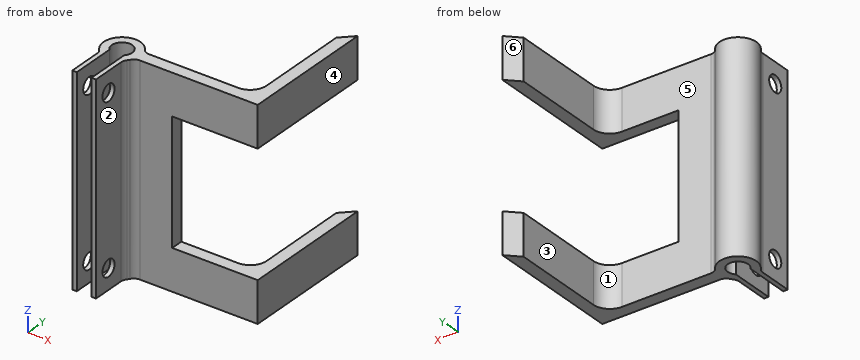
```python
from build123d import *

# Parameters (mm, degrees)
SKETCH_1_R          = 2.25
SKETCH_1_R_2        = 1.25
EXTRUDE_1_DEPTH     = 25
EXTRUDE_START       = -25
EXTRUDE_2_DEPTH     = 25
CUT_EXTRUDE_1_DEPTH = 25
SKETCH_4_W          = 0.55
SKETCH_4_H          = 25
EXTRUDE_3_DEPTH     = 2
EXTRUDE_4_DEPTH     = 25
FILLET_1_R          = 1
SKETCH_6_W          = 1.5
SKETCH_6_H          = 25
EXTRUDE_6_DEPTH     = 15
SKETCH_7_W          = 17.879358453
SKETCH_7_H          = 15
CUT_EXTRUDE_2_DEPTH = 50
FILLET_2_R          = 2
SKETCH_8_R          = 1
CUT_EXTRUDE_3_DEPTH = 10
CHAMFER_1_SIZE      = 1.5


with BuildPart() as part:
    # 草图1 → 凸台-拉伸1 (new body)
    with BuildSketch(Plane.XY):
        Circle(SKETCH_1_R)
        Circle(SKETCH_1_R_2, mode=Mode.SUBTRACT)
    extrude(amount=EXTRUDE_1_DEPTH)

    # 草图2 → 凸台-拉伸2 (add)
    with BuildSketch(Plane.XY.offset(25).offset(EXTRUDE_START)):
        with BuildLine():
            Line((-0.9, -4.25), (-0.9, -2.062159063))
            ThreePointArc((-0.9, -2.062159063), (-1.187355759, -1.911200225), (-1.45, -1.720465053))
            Line((-1.45, -1.720465053), (-1.45, -4.25))
            Line((-1.45, -4.25), (-0.9, -4.25))
        make_face()
        with BuildLine():
            ThreePointArc((1.45, -1.720465053), (1.187355759, -1.911200225), (0.9, -2.062159063))
            Line((0.9, -2.062159063), (0.9, -4.25))
            Line((0.9, -4.25), (1.45, -4.25))
            Line((1.45, -4.25), (1.45, -1.720465053))
        make_face()
    extrude(amount=EXTRUDE_2_DEPTH)

    # 草图3 → 切除-拉伸1 (cut)
    with BuildSketch(Plane.XY.offset(25)):
        Polygon((-0.9, -2.062159063), (-0.9, -0.608172981), (0.9, -0.572608175), (0.9, -2.062159063), (-0.22034315, -2.711539451), align=None)
    extrude(amount=-CUT_EXTRUDE_1_DEPTH, mode=Mode.SUBTRACT)

    # 草图4 → 凸台-拉伸3 (add)
    with BuildSketch(Plane.XZ.offset(4.25)):
        with Locations((1.175, 12.5)):
            Rectangle(SKETCH_4_W, SKETCH_4_H)
        with Locations((-1.175, 12.5)):
            Rectangle(SKETCH_4_W, SKETCH_4_H)
    extrude(amount=EXTRUDE_3_DEPTH)

    # 草图5 → 凸台-拉伸4 (add)
    with BuildSketch(Plane.XY.offset(25).offset(EXTRUDE_START)):
        with BuildLine():
            Line((2.121320344, 0.75), (17.121320344, 0.75))
            Line((17.121320344, 0.75), (17.121320344, -0.75))
            Line((17.121320344, -0.75), (2.121320344, -0.75))
            ThreePointArc((2.121320344, -0.75), (2.25, 0), (2.121320344, 0.75))
        make_face()
    extrude(amount=EXTRUDE_4_DEPTH)

    # 圆角1
    fillet_1_edges = [part.edges().sort_by_distance(p)[0] for p in [
        (-1.45, -1.720465053, 12.5),
        (1.45, -1.720465053, 12.5),
        (2.121320344, -0.75, 12.5),
        (2.121320344, 0.75, 12.5),
    ]]
    fillet(fillet_1_edges, radius=FILLET_1_R)

    # 草图6 → 凸台-拉伸6 (add)
    with BuildSketch(Plane(origin=(0, 0.75, 0), x_dir=(1, 0, 0), z_dir=(0, 1, 0))):
        with Locations((16.371320344, -12.5)):
            Rectangle(SKETCH_6_W, SKETCH_6_H)
    extrude(amount=EXTRUDE_6_DEPTH)

    # 草图7 → 切除-拉伸2 (cut, symmetric)
    with BuildSketch(Plane(origin=(0, 0.75, 0), x_dir=(1, 0, 0), z_dir=(0, 1, 0))):
        with Locations((15.621320344, -12.5)):
            Rectangle(SKETCH_7_W, SKETCH_7_H)
    extrude(amount=CUT_EXTRUDE_2_DEPTH, both=True, mode=Mode.SUBTRACT)

    # 圆角2
    fillet_2_edges = [part.edges().sort_by_distance(p)[0] for p in [
        (15.621320344, 0.75, 2.5),
        (15.621320344, 0.75, 22.5),
    ]]
    fillet(fillet_2_edges, radius=FILLET_2_R)

    # 草图8 → 切除-拉伸3 (cut)
    with BuildSketch(Plane.ZY.offset(1.45)):
        with Locations((2.5, -4.192707825)):
            Circle(SKETCH_8_R)
        with Locations((22.5, -4.192707825)):
            Circle(SKETCH_8_R)
    extrude(amount=-CUT_EXTRUDE_3_DEPTH, mode=Mode.SUBTRACT)

    # 倒角1
    chamfer_1_edges = [part.edges().sort_by_distance(p)[0] for p in [
        (15.621320344, 15.75, 2.5),
        (15.621320344, 15.75, 22.5),
    ]]
    chamfer(chamfer_1_edges, length=CHAMFER_1_SIZE - 0.0001)  # a hair under: the kernel refuses the full size


solid = part.part
```
Check sheet for the modelled part. Datum: model origin and axes. Units: mm. Face numbers are marked on the shaded views. A direction names the side the tool comes from. Round coordinates to 2 decimals unless told otherwise and drop trailing zeros. Order: outer loops, then holes, each group sorted by start corner. A loop starts at its lowest first (then second) coordinate and runs counter-clockwise, first axis right, second up.
1) Section check D-D (z = 17.75). Record the boundary of the cut face in (x, y).
2) Tool access check on the marked faces 1, 2 and 3. Record the directions out of +Z, -Z, +X, -X, +Y, -Y that give a thin tool (end or side, any length) a straight path to the whole face; none if there is none.
3) Section check C-C (x = 12). Record the boundary of the cut face in (y, z).
4) Mould release check, pull along X, two halves, no side actions. Record for the marked faces 4, 5 and 6: +X half, -X half, draft (parallel to the pull), parting line (faces both ways), or undercut.
5) Section check B-B (y = 0). Record the boundary of the cut face in (x, z), and give its area (3 significant figures).
6) Go/stop test with flat-tipped pins: pin 1 Ø2 at (x, y) = (0, 0) entering from +Z; pin 2 Ø3 at (x, z) = (5.5, 14.5) entering from +Y; pin 3 Ø2.5 at (y, z) = (10, 2.5) entering from -X; pin 4 Ø4.5 at (y, z) = (-4.5, 12.5) entering from -X. Record where each tip stops, or that it passes through.
7) Scan lines: line 1 (Z direction, x = 11.25, y = -0.5); line 2 (X direction, y = 3, z = 4.75); line 3 (Y direction, x = 1.1, z = 2.5). Record each from-to range of solid material in increasing order.
8) Section check A-A (z = 22.5). Give the number of separate pieces and of enclosed holes in the cut face, and give its area (3 significant figures).
Result:
1. outline: (-1.7, -1.48) arc R1 cw to (-1.45, -2.14) - (-1.45, -6.25) - (-0.9, -6.25) - (-0.9, -0.87) arc R1.25 cw (long way) to (0.9, -0.87) - (0.9, -6.25) - (1.45, -6.25) - (1.45, -2.14) arc R1 cw to (1.7, -1.48) arc R2.25 ccw to (1.9, -1.21) arc R1 cw to (2.74, -0.75) - (6.68, -0.75) - (6.68, 0.75) - (2.74, 0.75) arc R1 cw to (1.9, 1.21) arc R2.25 ccw (long way) to start
2. face 1: +Z, -Z, +Y
2. face 2: +Z, -Z, +X, -Y
2. face 3: +Z, -Z, -X, +Y
3. outline: (-0.75, 0) - (0.75, 0) - (0.75, 5) - (-0.75, 5) - close; (-0.75, 20) - (0.75, 20) - (0.75, 25) - (-0.75, 25) - close
4. face 4: +X half
4. face 5: undercut
4. face 6: -X half
5. outline: (-2.25, 0) - (-1.25, 0) - (-1.25, 25) - (-2.25, 25) - close; (1.25, 0) - (17.12, 0) - (17.12, 5) - (6.68, 5) - (6.68, 20) - (17.12, 20) - (17.12, 25) - (1.25, 25) - close
5. area: 265 mm2
6. pin 1: passes through
6. pin 2: stops at y = 0.75
6. pin 3: stops at x = 15.62
6. pin 4: stops at x = -1.45
7. line 1: z = 0 to 5, 20 to 25
7. line 2: x = 15.62 to 17.12
7. line 3: y = -6.25 to -5.19, -3.19 to -0.59, 0.59 to 1.96
8. separate pieces: 3
8. enclosed holes: 0
8. area: 56.4 mm2
